The listing builds one solid part. Answer for the finished solid, in the listing's coordinates (mm). A direction names the side the tool comes from. Coordinates: 2 decimals unless noted, no trailing zeros. Loops run counter-clockwise (first coordinate to the right, second up) from the corner with the lowest first, then second, coordinate; pieces in that order, holes last. Notation, with made-up numbers: (-2.75, -25) - (37.25, -25) arc R26 ccw to (37.25, -7) - close; hole circle Ø4 at (80, 61). An arc over 180 degrees is marked (long way). Return JSON: item names as keys, results as strings. Group by question number.
1. Section A-A (y = 44.5) is taken. Write down the section's boundary in (x, z).
2. Find the intervals of material crossed by line 1 along Y through (x, z) = (33, 16); line 2 along Y through (x, z) = (42, 29.5), in increasing order.
3. The mould has two halves that part along X. Classify faces 1 (the face through (0.8, 36.8, 33.02)), 2 (the face through (30, 2.54, 15)), 3 (the face through (50.8, 25, 16)): pulls with the +X half, pulls with the -X half, needs draft (parallel to the pull), parting line crosses it, or undercut.
4. Which of the six approach directions +Z, -Z, +X, -X, +Y, -Y give full straight-line access (tool end or side, diameter ignored) to faces 4 (the face through (0, 25, 16)), 5 (the face through (6.87, 1.25, 23.38)), 6 (the face through (25, 49.784, 30))?
5. This flat-tipped pin is pushed along its axis until it touches: P1, Ø23, axis at x = 15.5, y = 20, coming from the +Z side. Where does it stop, or does it pass through?
```python
from build123d import *

# Parameters (mm, degrees)
F0_W     = 50.8
F0_H     = 50.8
F1_DEPTH = 2.54
F2_W     = 50.8
F2_H     = 50.8
F2_W_2   = 48.768
F2_H_2   = 48.768
F3_DEPTH = 30.48
F4_W     = 50.8
F4_H     = 50.8
F4_W_2   = 48.768
F4_H_2   = 48.768
F4_W_3   = 45.72
F4_H_3   = 45.72
F5_DEPTH = 25.4
F6_R     = 10.16
F7_DEPTH = 25.4


with BuildPart() as f1:
    # F0 (on Top) → F1 (new body)
    with BuildSketch(Plane.XY):
        with Locations((25.4, 25.4)):
            Rectangle(F0_W, F0_H)
    extrude(amount=F1_DEPTH)

    # F2 (on face) → F3 (join)
    with BuildSketch(Plane.XY.offset(2.54)):
        with Locations((25.4, 25.4)):
            Rectangle(F2_W, F2_H)
        with Locations((25.4, 25.4)):
            Rectangle(F2_W_2, F2_H_2, mode=Mode.SUBTRACT)
    extrude(amount=F3_DEPTH)

    # F4 (on face) → F5 (join)
    with BuildSketch(Plane.XY.offset(2.54)):
        with Locations((25.4, 25.4)):
            Rectangle(F4_W, F4_H)
        with Locations((25.4, 25.4)):
            Rectangle(F4_W_2, F4_H_2, mode=Mode.SUBTRACT)
        with Locations((25.4, 25.4)):
            Rectangle(F4_W_2, F4_H_2)
        with Locations((25.4, 25.4)):
            Rectangle(F4_W_3, F4_H_3, mode=Mode.SUBTRACT)
    extrude(amount=F5_DEPTH)

    # F6 (on face) → F7 (cut)
    with BuildSketch(Plane.XZ):
        with Locations((14.354912, 16.51)):
            Circle(F6_R)
    extrude(amount=-F7_DEPTH, mode=Mode.SUBTRACT)


solid = f1.part
```
The answers:
{
 "1": {"outline": "(0, 0) - (50.8, 0) - (50.8, 33.02) - (49.78, 33.02) - (49.78, 27.94) - (48.26, 27.94) - (48.26, 2.54) - (2.54, 2.54) - (2.54, 27.94) - (1.02, 27.94) - (1.02, 33.02) - (0, 33.02) - close"},
 "2": {"line 1": "y = 0 to 2.54, 48.26 to 50.8", "line 2": "y = 0 to 1.02, 49.78 to 50.8"},
 "3": {"face 1": "needs draft", "face 2": "undercut", "face 3": "pulls with the +X half"},
 "4": {"face 4": "+Z, -Z, -X, +Y, -Y", "face 5": "-Y", "face 6": "+Z"},
 "5": {"P1": "stops at z = 2.54"}
}
